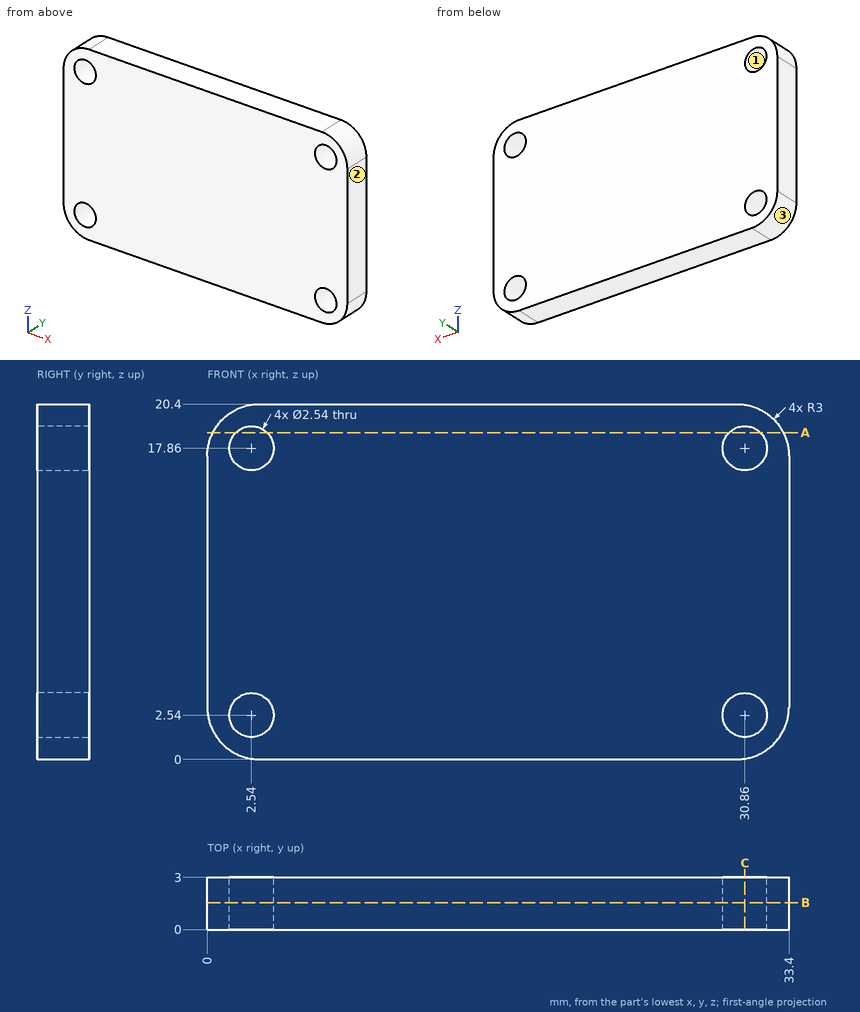
Answer from the drawing. Dimensions are ordinates in mm from the lowest x, y and z of the part. Coordinates: 2 decimals unless noted, no trailing zeros. Loops run counter-clockwise (first coordinate to the right, second up) from the corner with the lowest first, then second, coordinate; pieces in that order, holes last. Notation, with made-up numbers: (44, -20) -> (72, -20) arc R23 ccw to (72, -7) -> close; hole circle Ø5 at (9.25, 31.5). An arc over 180 degrees is marked (long way). Answer as CSV lines item,"result".
Q1. The part is cut by section A-A on z = 18.75. Write down the section's boundary in (x, y).
Findings:
outline,"(0.32, 0) -> (1.63, 0) -> (1.63, 3) -> (0.32, 3) -> close; (3.45, 0) -> (29.95, 0) -> (29.95, 3) -> (3.45, 3) -> close; (31.77, 0) -> (33.08, 0) -> (33.08, 3) -> (31.77, 3) -> close"
Q2. Find the intervals of material crossed by probe 1 along X at (y, z) = (1.5, 17.86); probe 2 along Z at (x, y) = (30, 0.15), in increasing order.
Findings:
probe 1,"x = 0.04 to 1.27, 3.81 to 29.59, 32.13 to 33.36"
probe 2,"z = 0 to 1.61, 3.47 to 16.93, 18.79 to 20.4"
Q3. The part is cut by section B-B on y = 1.55. Write down the section's boundary in (x, z), and give its area (3 significant figures).
Findings:
outline,"(0, 3) arc R3 ccw to (3, 0) -> (30.4, 0) arc R3 ccw to (33.4, 3) -> (33.4, 17.4) arc R3 ccw to (30.4, 20.4) -> (3, 20.4) arc R3 ccw to (0, 17.4) -> close; hole circle Ø2.54 at (2.54, 2.54); hole circle Ø2.54 at (2.54, 17.86); hole circle Ø2.54 at (30.86, 2.54); hole circle Ø2.54 at (30.86, 17.86)"
area,"653 mm²"
Q4. The part is cut by section C-C on x = 30.86. Write down the section's boundary in (y, z).
Findings:
outline,"(0, 0.04) -> (3, 0.04) -> (3, 1.27) -> (0, 1.27) -> close; (0, 3.81) -> (3, 3.81) -> (3, 16.59) -> (0, 16.59) -> close; (0, 19.13) -> (3, 19.13) -> (3, 20.36) -> (0, 20.36) -> close"
Q5. For a pull along Z with two mould halves and no side action, classify the marked faces 1, 2 and 3 as +Z half, -Z half, draft (parallel to the pull), parting line (faces both ways), or undercut.
Findings:
face 1,"undercut"
face 2,"draft"
face 3,"-Z half"
